Drawing for the job (mm, zero at the part's lowest x, y, z). A direction names the side the tool comes from. Give positions to 0.01 mm unless a question says otherwise; leave off trailing zeros. Loops run counter-clockwise (first coordinate to the right, second up) from the corner with the lowest first, then second, coordinate; pieces in that order, holes last.
1) Two-plate mould, pull along Y, no slides. Class the marked faces 1, 2 and 3: +Y half, -Y half, draft (parallel to the pull), parting line (faces both ways), or undercut.
2) Band-saw the part on C-C on z = 1.75. List the corners of the cut face in (x, y).
3) Band-saw the part on D-D on z = 14. List the corners of the cut face in (x, y), then the cut area to 3 significant figures.
4) 3-axis set-ups, long thin cutter, end or side, ignore diameter. For the marked faces 4, 5 and 6: which of +Z, -Z, +X, -X, +Y, -Y reach the whole face in a straight line?
5) Flat gauge pins, fed straight in: P1, Ø2.5, axis at x = 9, y = 73, coming from the +Z side; P2, Ø4, axis at x = 44.5, y = 35, coming from the +Z side; P3, Ø10, axis at x = 20, y = 17.5, coming from the -Z side; P4, Ø2.5, axis at y = 72, z = 23, coming from the -X side. Where does each tip first touch, or does it go through?
6) Wall check: line 1 (Y direction, x = 25.4, z = 4.5); line 2 (Y direction, x = 13.5, z = 18); line 3 (Z direction, x = 37, y = 57.5). Give the ranges that are in metal, low to high.
7) Band-saw the part on B-B on y = 33. List the corners of the cut face in (x, z), then the cut area to 3 significant figures.
8) Band-saw the part on A-A on x = 25.4. List the corners of the cut face in (y, z), then the cut area to 3 significant figures.
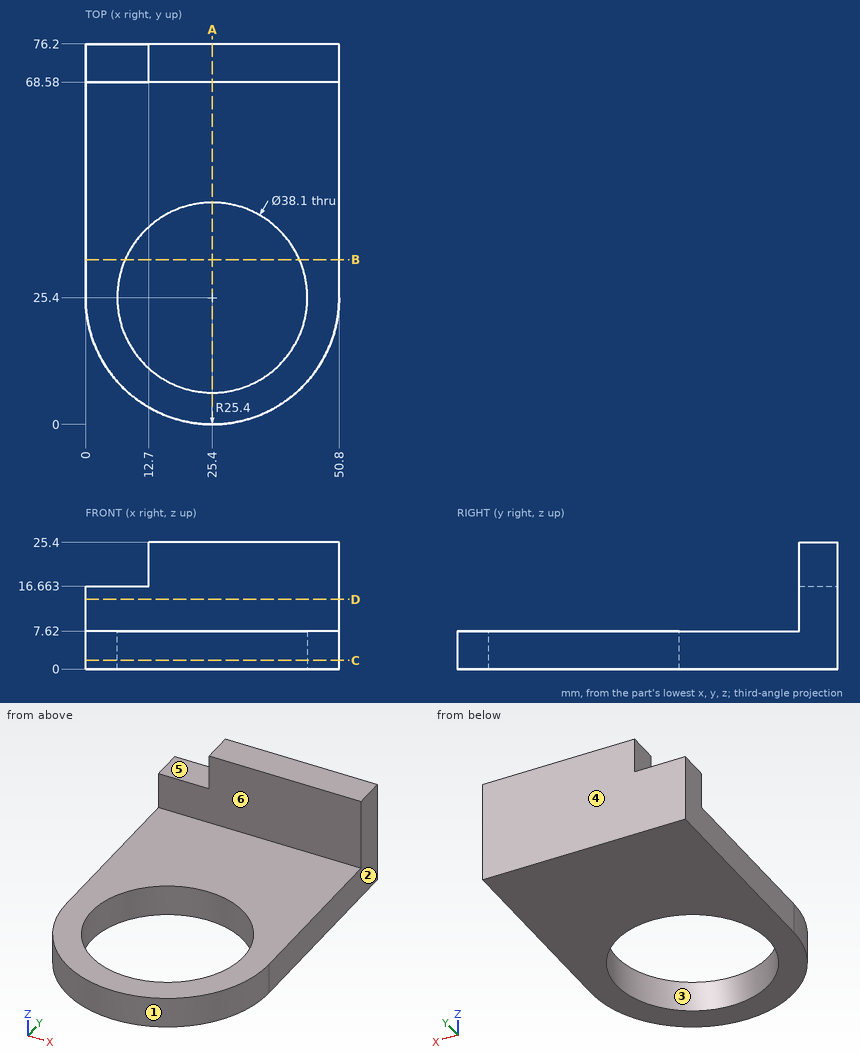
Findings below:
1. face 1: -Y half
1. face 2: draft
1. face 3: undercut
2. outline: (0, 25.4) arc R25.4 ccw to (50.8, 25.4) - (50.8, 76.2) - (0, 76.2) - close; hole circle Ø38.1 at (25.4, 25.4)
3. outline: (0, 68.58) - (50.8, 68.58) - (50.8, 76.2) - (0, 76.2) - close
3. area: 387 mm2
4. face 4: +Z, -Z, +X, -X, +Y
4. face 5: +Z, -X, +Y, -Y
4. face 6: +Z, +X, -X, -Y
5. P1: stops at z = 16.66
5. P2: stops at z = 7.62
5. P3: passes through
5. P4: stops at x = 12.7
6. line 1: y = 0 to 6.35, 44.45 to 76.2
6. line 2: y = 68.58 to 76.2
6. line 3: z = 0 to 7.62
7. outline: (0, 0) - (7.93, 0) - (7.93, 7.62) - (0, 7.62) - close; (42.87, 0) - (50.8, 0) - (50.8, 7.62) - (42.87, 7.62) - close
7. area: 121 mm2
8. outline: (0, 0) - (6.35, 0) - (6.35, 7.62) - (0, 7.62) - close; (44.45, 0) - (76.2, 0) - (76.2, 25.4) - (68.58, 25.4) - (68.58, 7.62) - (44.45, 7.62) - close
8. area: 426 mm2
